The model under review builds one solid part; all positions refer to its coordinate system, in mm. Face numbers are marked on the shaded views. A direction names the side the tool comes from. Round coordinates to 2 decimals unless told otherwise and drop trailing zeros. Order: outer loops, then holes, each group sorted by start corner. A loop starts at its lowest first (then second) coordinate and runs counter-clockwise, first axis right, second up.
Autodesk Inventor part; units mm, degrees
ref_plane "РабПлоскость2" through (-21.3726, 0, 0) normal (1, 0, 0) x (0, 0, -1)
ref_plane "YZ Plane" through (0, 0, 0) normal (1, 0, 0) x (0, 1, 0)
ref_plane "XZ Plane" through (0, 0, 0) normal (0, 1, 0) x (-1, 0, 0)
sketch "Эскиз1" plane through (0, 0, 0) normal (0, 0, 1) x (1, 0, 0)
  line L0 (0, 0) -> (-21.3726, 0)
  arc A0 (-19, 1.9227) -> (-21, 2.2534) centre (-20.0273, 1.9227) ccw
  line L1 (-19, 1.9227) -> (-19, 1.45)
  line L2 (-19, 1.45) -> (0, 1.45)
  line L3 (0, 1.45) -> (0, 0)
  line L4 (-21.6724, 2.95) -> (-19.1128, 2.95)
  arc A1 (-21, 2.2534) -> (-21.3726, 0) centre (-14.3726, 0) ccw
  dimension "d0" = 2.9
  dimension "d1" = 5.9
  dimension "d2" = 2
  dimension "d3" = 19
  dimension "d4" = 7
revolve "Вращение1" add sketch "Эскиз1" angle 360 about axis through (0, 0, 0) along (-1, 0, 0)
chamfer "Фаска1" distance 0.3 angle 45 1 edges at (0, -1.45, 0)
ref_plane "РабПлоскость2" through (-21.3726, 0, 0) normal (1, 0, 0) x (0, 0, -1)
sketch "Эскиз2" plane through (-21.3726, 0, 0) normal (1, 0, 0) x (0, 0, -1)
  line L0 (-0.4, 1.5) -> (0.4, 1.5)
  line L1 (0.4, 1.5) -> (0.4, -1.5)
  line L2 (0.4, -1.5) -> (-0.4, -1.5)
  line L3 (-0.4, -1.5) -> (-0.4, 1.5)
  line L4 (-1.5, 0.4) -> (1.5, 0.4)
  line L5 (1.5, 0.4) -> (1.5, -0.4)
  line L6 (1.5, -0.4) -> (-1.5, -0.4)
  line L7 (-1.5, -0.4) -> (-1.5, 0.4)
  point P0 (0, 0)
  point P1 (0, 1.5)
  point P2 (0, 0.4)
  point P3 (-1.5, 0)
  point P4 (-0.4, 0)
  point P5 (0.4, 0.4)
  point P6 (-0.4, 0.4)
  point P7 (-0.4, -0.4)
  point P8 (0.4, -0.4)
  dimension "d10" = 0.8
  dimension "d11" = 3
extrude "Выдавливание1" cut sketch "Эскиз2" along normal blind 1.2
properties part number "Винт М3х19"
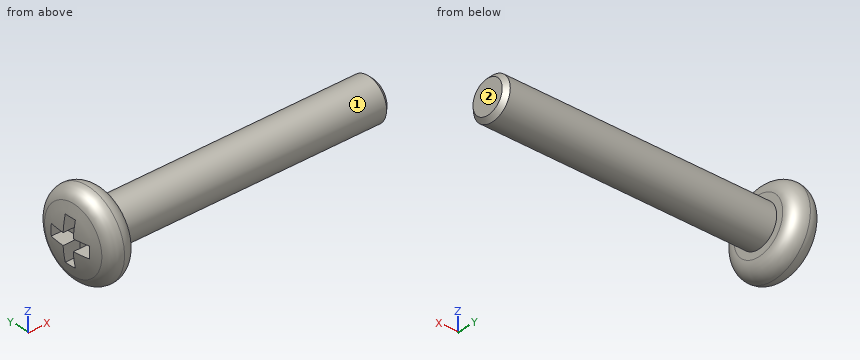
(1) To check wall thickness, follow L1, parallel to Z at x = -1.25, y = -0.1; L2, parallel to X at y = 0.3, z = 0.4; L3, parallel to Y at x = -19.25, z = -2.25. State the ranges of each line that lie inside material, in increasing order.
(2) We need section A-A (x = -13). Give the boundary of the cut face in (y, z), and give its area (3 significant figures).
(3) Tool access review of the marked faces 1 and 2: name each direction out of +Z, -Z, +X, -X, +Y, -Y from which nothing blocks a thin tool from reaching the whole face with its end or side.
(4) Clearance check with flat-ended pins moving along their axes: P1, Ø1, axis at y = 2, z = -0.5, coming from the -X side; P2, Ø0.9, axis at x = -21, z = 0, coming from the +Y side; P3, Ø0.9, axis at x = -21, y = -1, coming from the -Z side. State where each tip first meets the part, or that it passes through.
Verdict:
1. L1: z = -1.45 to 1.45
1. L2: x = -20.17 to 0
1. L3: y = -1.29 to 1.29
2. outline: circle Ø2.9 at (0, 0)
2. area: 6.61 mm2
3. face 1: +X
3. face 2: +Z, -Z, +X, +Y, -Y
4. P1: stops at x = -21.2
4. P2: stops at y = 2.81
4. P3: stops at z = -2.66
